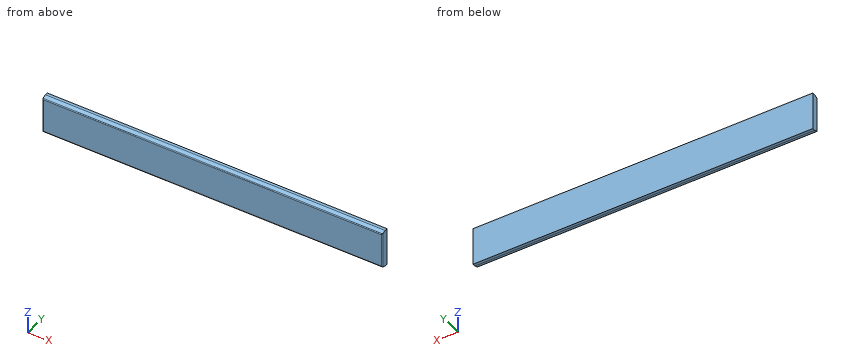
```python
from build123d import *

# Parameters (mm, degrees)
F0_W     = 1828.8
F0_H     = 203.2
F1_DEPTH = 38.1
F2_SIZE2 = 8.3203595553
F2_SIZE  = 22.86
F3_SIZE2 = 8.3203595553
F3_SIZE  = 22.86
F4_R     = 5.08


with BuildPart() as f1:
    # F0 (on Front) → F1 (new body)
    with BuildSketch(Plane.XZ):
        with Locations((-47.5488106235, 0)):
            Rectangle(F0_W, F0_H)
    extrude(amount=F1_DEPTH)

    # F2
    f2_edges = [f1.edges().sort_by_distance(p)[0] for p in [
        (-47.548811, -38.1, 101.6),
    ]]
    f2_side = f1.faces().sort_by_distance((-47.548811, -19.05, 101.6))[0]
    chamfer(f2_edges, length=F2_SIZE, length2=F2_SIZE2, reference=f2_side)

    # F3
    f3_edges = [f1.edges().sort_by_distance(p)[0] for p in [
        (-47.548811, -38.1, -101.6),
    ]]
    f3_side = f1.faces().sort_by_distance((-47.548811, -19.05, -101.6))[0]
    chamfer(f3_edges, length=F3_SIZE, length2=F3_SIZE2, reference=f3_side)

    # F4
    f4_edges = [f1.edges().sort_by_distance(p)[0] for p in [
        (-961.948811, -38.1, 0),
        (-47.548811, -38.1, -93.27964),
        (-47.548811, -38.1, 93.27964),
        (866.851189, -38.1, 0),
    ]]
    fillet(f4_edges, radius=F4_R)


solid = f1.part
```
Could you check a few things on this model? Use its own coordinates, in mm. Coordinates: 2 decimals unless noted, no trailing zeros. Loops run counter-clockwise (first coordinate to the right, second up) from the corner with the lowest first, then second, coordinate; pieces in that order, holes last. Notation, with made-up numbers: M 51.5,40.5 L 77.5,40.5 A23 ccw 77.5,50.5 Z; hole C -22.75,5.25 d1. An arc over 180 degrees is marked long. Put each result on its own line as item: value. Start each with the question number.
(1) Will these pins go through, and if not, where does the flat tip stop? P1, Ø2, axis at x = -310.5, z = 63, coming from the +Y side; P2, Ø1.5, axis at x = 252.5, y = -19, coming from the -Z side; P3, Ø2, axis at y = -34.5, z = 57, coming from the -X side.
(2) I need wall thicknesses on line 1 (Z direction, x = -455.5, y = -34); line 2 (Z direction, x = -426, y = -33.5). Which ranges of each line are inside material? Lowest first, please. Write a range as from..to.
(3) Suppose I cut it at A-A on x = 537. Please give me the cut outline in (y, z).
(4) Suppose I cut it at B-B on y = -21. Please give me the cut outline in (x, z).
Solutions:
1. P1: stops at y = 0
1. P2: stops at z = -100.5
1. P3: stops at x = -961.93
2. line 1: z = -94.77..94.77
2. line 2: z = -94.95..94.95
3. outline: M -38.1,-89.72 A5.08 ccw -34.76,-94.5 L -15.24,-101.6 L 0,-101.6 L 0,101.6 L -15.24,101.6 L -34.76,94.5 A5.08 ccw -38.1,89.72 Z
4. outline: M -961.95,-99.5 L 866.85,-99.5 L 866.85,99.5 L -961.95,99.5 Z
